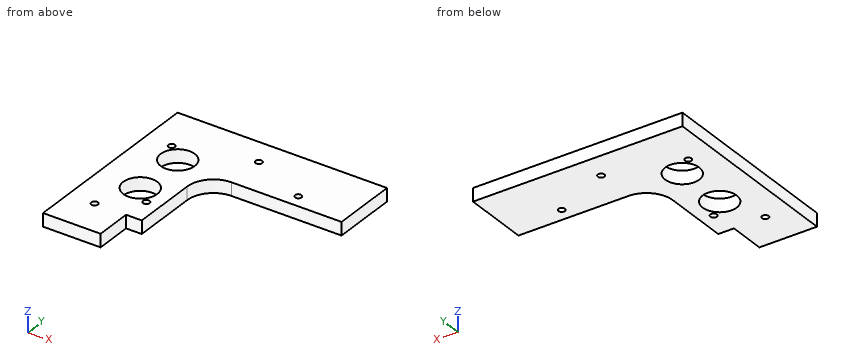
```python
from build123d import *

# Parameters (mm, degrees)
F1_DEPTH = 6.35
F2_R     = 1.5875
F2_R_2   = 8.255
F3_DEPTH = 6.35
F4_W     = 101.6
F4_H     = 93.98
F5_DEPTH = 25.4


with BuildPart() as f1:
    # F0 (on Top) → F1 (new body)
    with BuildSketch(Plane.XY):
        with BuildLine():
            Line((0, 93.98), (0, 0))
            Line((0, 0), (27.94, 0))
            Line((27.94, 0), (27.94, 17.78))
            Line((27.94, 17.78), (35.56, 17.78))
            Line((35.56, 17.78), (35.56, 49.53))
            ThreePointArc((35.56, 49.53), (39.279744, 58.510256), (48.26, 62.23))
            Line((48.26, 62.23), (154.94, 62.23))
            ThreePointArc((154.94, 62.23), (163.920256, 58.510256), (167.64, 49.53))
            Line((167.64, 49.53), (167.64, 17.78))
            Line((167.64, 17.78), (175.26, 17.78))
            Line((175.26, 17.78), (175.26, 0))
            Line((175.26, 0), (203.2, 0))
            Line((203.2, 0), (203.2, 93.98))
            Line((203.2, 93.98), (0, 93.98))
        make_face()
    extrude(amount=F1_DEPTH)

    # F2 (on face) → F3 (cut)
    with BuildSketch(Plane.XY.offset(6.35)):
        with Locations((12.7, 17.78)):
            Circle(F2_R)
        with Locations((28.956, 30.48)):
            Circle(F2_R)
        with Locations((20.828, 37.973)):
            Circle(F2_R_2)
        with Locations((20.828, 64.135)):
            Circle(F2_R_2)
        with Locations((12.7, 71.628)):
            Circle(F2_R)
        with Locations((48.26, 81.28)):
            Circle(F2_R)
        with Locations((76.2, 68.58)):
            Circle(F2_R)
        with Locations((127, 68.58)):
            Circle(F2_R)
        with Locations((154.94, 81.28)):
            Circle(F2_R)
        with Locations((174.244, 71.628)):
            Circle(F2_R)
        with Locations((182.372, 64.135)):
            Circle(F2_R_2)
        with Locations((182.372, 37.973)):
            Circle(F2_R_2)
        with Locations((190.5, 30.48)):
            Circle(F2_R)
        with Locations((190.5, 17.78)):
            Circle(F2_R)
    extrude(amount=-F3_DEPTH, mode=Mode.SUBTRACT)

    # F4 (on Top) → F5 (cut)
    with BuildSketch(Plane.XY):
        with Locations((152.4, 46.99)):
            Rectangle(F4_W, F4_H)
    extrude(amount=F5_DEPTH, mode=Mode.SUBTRACT)


solid = f1.part
```
Source: CAD feature listing. Evaluate the final solid. Frame: model axes, mm. Round coordinates to 2 decimals unless told otherwise and drop trailing zeros. Loops run counter-clockwise (first coordinate to the right, second up) from the corner with the lowest first, then second, coordinate; pieces in that order, holes last. Notation, with made-up numbers: (56.25, 74.25) - (103.25, 74.25) arc R38 ccw to (103.25, 113.25) - close; hole circle Ø3 at (11, 50). An arc over 180 degrees is marked (long way). Use CSV: the item, a comma, the result in double quotes.
Q1. Ray query, line 1 along Y through (x, z) = (48.26, 4.25); line 2 along Y through (x, z) = (52, 1); line 3 along X through (y, z) = (68, 5). Return the intervals inside material, ascending.
Reported:
line 1,"62.23 to 79.69, 82.87 to 93.98"
line 2,"62.23 to 93.98"
line 3,"0 to 13.53, 28.12 to 74.72, 77.68 to 101.6"
Q2. Section query B-B, the plane y = 81.28. Output: boundary loops of the cut face in (x, z), then the cut area to 3 significant figures.
Reported:
outline,"(0, 0) - (46.67, 0) - (46.67, 6.35) - (0, 6.35) - close; (49.85, 0) - (101.6, 0) - (101.6, 6.35) - (49.85, 6.35) - close"
area,"625 mm^2"
Q3. Section query C-C, the plane z = 2.75. Output: boundary loops of the cut face in (x, y) (1 decimal), then the cut area to 3 significant figures.
Reported:
outline,"(0, 0) - (27.9, 0) - (27.9, 17.8) - (35.6, 17.8) - (35.6, 49.5) arc R12.7 cw to (48.3, 62.2) - (101.6, 62.2) - (101.6, 94) - (0, 94) - close; hole circle Ø3.2 at (12.7, 17.8); hole circle Ø3.2 at (12.7, 71.6); hole circle Ø16.5 at (20.8, 38); hole circle Ø16.5 at (20.8, 64.1); hole circle Ø3.2 at (29, 30.5); hole circle Ø3.2 at (48.3, 81.3); hole circle Ø3.2 at (76.2, 68.6)"
area,"4,870 mm^2"
Q4. Section query A-A, the plane x = 76.2. Output: boundary loops of the cut face in (y, z), then the cut area to 3 significant figures.
Reported:
outline,"(62.23, 0) - (66.99, 0) - (66.99, 6.35) - (62.23, 6.35) - close; (70.17, 0) - (93.98, 0) - (93.98, 6.35) - (70.17, 6.35) - close"
area,"181 mm^2"
Q5. Pin query (flat end, axial travel): pin 1 Ø13 at (x, y) = (20.828, 37.973) entering from +Z; pin 2 Ø1.9 at (y, z) = (34, 1.5) entering from +X; pin 3 Ø1.9 at (x, z) = (33, 2) entering from -Y. Return the tip coordinate at first contact, or that it passes through.
Reported:
pin 1,"through"
pin 2,"x = 35.56"
pin 3,"y = 17.78"
Q6. Section query D-D, the plane x = 88.5. Output: boundary loops of the cut face in (y, z), then the cut area to 3 significant figures.
Reported:
outline,"(62.23, 0) - (93.98, 0) - (93.98, 6.35) - (62.23, 6.35) - close"
area,"202 mm^2"
